```python
from build123d import *

# Parameters (mm, degrees)
SKETCH1_W           = 250
SKETCH1_H           = 200
BOSS_EXTRUDE1_DEPTH = 3
SKETCH2_W           = 220.76
SKETCH2_H           = 139
CUT_EXTRUDE1_DEPTH  = 321.170267202
SKETCH5_W           = 3
SKETCH5_H           = 20
CUT_EXTRUDE3_DEPTH  = 10


with BuildPart() as part:
    # Sketch1 → Boss-Extrude1 (new body)
    with BuildSketch(Plane.XY):
        with Locations((125, 100)):
            Rectangle(SKETCH1_W, SKETCH1_H)
    extrude(amount=BOSS_EXTRUDE1_DEPTH)

    # Sketch2 → Cut-Extrude1 (cut, through all)
    with BuildSketch(Plane.XY.offset(3)):
        with Locations((125, 115.88)):
            Rectangle(SKETCH2_W, SKETCH2_H)
    extrude(amount=-CUT_EXTRUDE1_DEPTH, mode=Mode.SUBTRACT)

    # Sketch5 → Cut-Extrude3 (cut)
    with BuildSketch(Plane.XY.offset(3)):
        with Locations((1.5, 20)):
            Rectangle(SKETCH5_W, SKETCH5_H)
        with Locations((248.5, 20)):
            Rectangle(SKETCH5_W, SKETCH5_H)
    extrude(amount=-CUT_EXTRUDE3_DEPTH, mode=Mode.SUBTRACT)


solid = part.part
```
Input: part model. Units: mm. Frame: model coordinates. Give positions to 0.01 mm unless a question says otherwise; leave off trailing zeros. Order: outer loops, then holes, each group sorted by start corner. A loop starts at its lowest first (then second) coordinate and runs counter-clockwise, first axis right, second up. Notation, with made-up numbers: M 65,-28.75 L 83,-28.75 A8 ccw 83,-15.75 Z; hole C 54.25,-4 d9. An arc over 180 degrees is marked long. Return JSON: item names as keys, results as strings.
Item 1: First-contact query: P1, Ø0.9, axis at y = 23.5, z = 2, coming from the +X side. Flat tip, straight axial feed; report the tip coordinate or a pass-through.
Solutions:
{"P1": "x = 247"}
Item 2: Cut plane C-C (y = 170). Return loops of the section in (x, z), then the cut area to 3 significant figures.
Solutions:
{"outline": "M 0,0 L 14.62,0 L 14.62,3 L 0,3 Z; M 235.38,0 L 250,0 L 250,3 L 235.38,3 Z", "area": "87.7 mm^2"}
Item 3: Ray query, probe 1 along Y at (x, z) = (196, 0.25); probe 2 along X at (y, z) = (110.5, 2.6); probe 3 along X at (y, z) = (13, 1.3). Return the intervals inside material, ascending.
Solutions:
{"probe 1": "0 to 46.38, 185.38 to 200", "probe 2": "0 to 14.62, 235.38 to 250", "probe 3": "3 to 247"}
Item 4: Cut plane B-B (x = 43). Return loops of the section in (y, z).
Solutions:
{"outline": "M 0,0 L 46.38,0 L 46.38,3 L 0,3 Z; M 185.38,0 L 200,0 L 200,3 L 185.38,3 Z"}
Item 5: Cut plane A-A (z = 1). Return loops of the section in (x, y).
Solutions:
{"outline": "M 0,0 L 250,0 L 250,10 L 247,10 L 247,30 L 250,30 L 250,200 L 0,200 L 0,30 L 3,30 L 3,10 L 0,10 Z; hole M 14.62,46.38 L 235.38,46.38 L 235.38,185.38 L 14.62,185.38 Z"}
Item 6: Cut plane D-D (y = 23). Return loops of the section in (x, z), then the cut area to 3 significant figures.
Solutions:
{"outline": "M 3,0 L 247,0 L 247,3 L 3,3 Z", "area": "732 mm^2"}
